Answer from the drawing. Dimensions are ordinates in mm from the lowest x, y and z of the part. A direction names the side the tool comes from. Give positions to 0.01 mm unless a question says otherwise; leave off trailing zeros. Write each loop counter-clockwise with the first axis right and the second up, starting at its lowest first coordinate (ties: lowest second). Pieces come first, ordered by that corner, then holes. Notation, with made-up numbers: (41, 13) -> (90, 13) arc R25 ccw to (90, 27) -> close; hole circle Ø4 at (-19, 52.25). An arc over 180 degrees is marked (long way). Use a Markdown table: item, result. Add a question column.
Q1. For the marked faces 3 and 4, determine the directions among +Z, -Z, +X, -X, +Y, -Y from which every point of the face is accessible in a straight line to the end or side of a thin tool.
Q2. Section D-D, the plane z = 36.5 is taken. Give the vertices of the cut face in (x, y).
Q3. Each of these flat-tipped pins is pushed along its axis until it touches: pin 1 Ø2.5 at (x, z) = (3.5, 25.5) entering from +Y; pin 2 Ø8 at (x, z) = (30.5, 22.5) entering from +Y; pin 3 Ø2 at (y, z) = (1, 36) entering from +X. Where does it stop, or does it pass through?
Q4. Section A-A, the plane x = 47.5 is taken. Give the vertices of the cut face in (y, z), plus the area to 3 significant figures.
Q5. For a pull along X with two mould halves and no side action, classify the marked faces 1 and 2 as pulls with the +X half, pulls with the -X half, needs draft (parallel to the pull), parting line crosses it, or undercut.
Q6. Section C-C, the plane y = 2 is taken. Give the vertices of the cut face in (x, z).
Q7. Consider line 1 (X direction, y = 3.1, z = 47.5); line 2 (X direction, y = 2.05, z = 22.5). Determine where each line is inside the solid, lowest interval first.
Q8. Section B-B, the plane z = 47.5 is taken. Give the vertices of the cut face in (x, y).
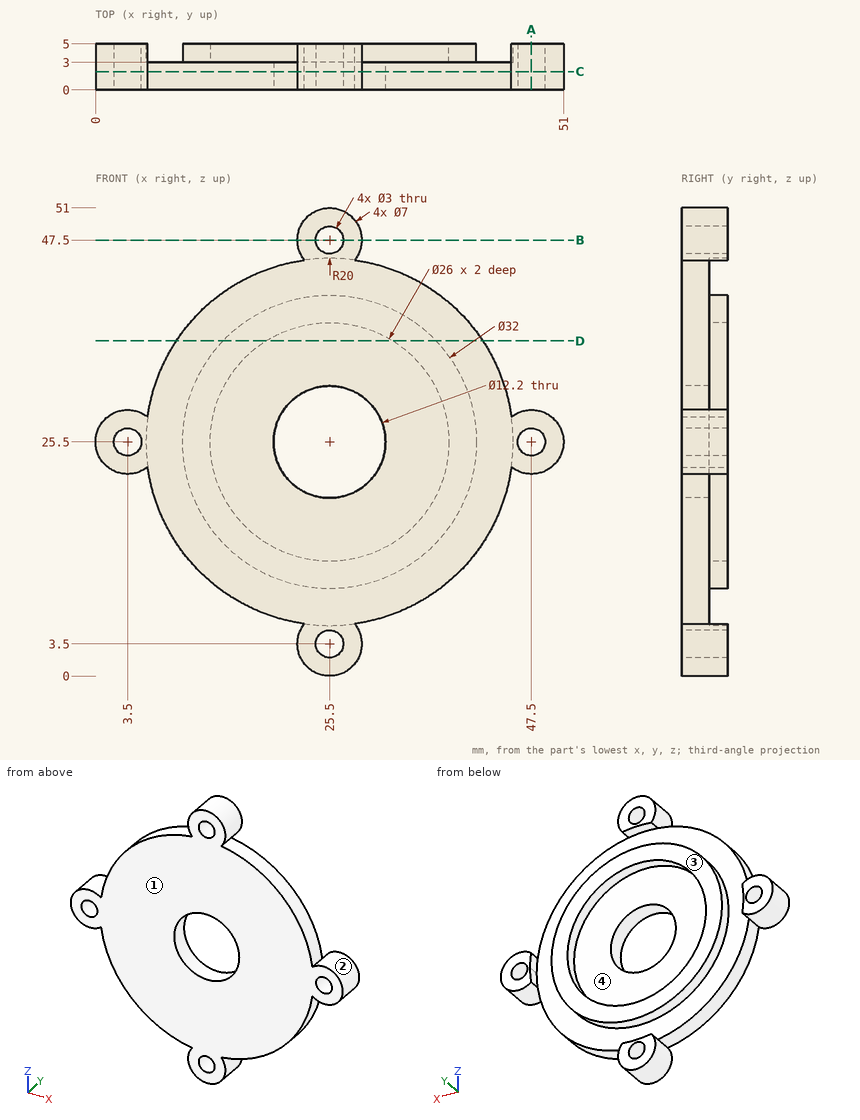
Result set:
| question | item | result |
|---|---|---|
| 1 | face 3 | +Z, -Z, +X, -X, +Y |
| 1 | face 4 | +Y |
| 2 | outline | (8.8, 0) -> (42.2, 0) -> (42.2, 3) -> (37.12, 3) -> (37.12, 5) -> (32.43, 5) -> (32.43, 3) -> (18.57, 3) -> (18.57, 5) -> (13.88, 5) -> (13.88, 3) -> (8.8, 3) -> close |
| 3 | pin 1 | passes through |
| 3 | pin 2 | stops at y = 3 |
| 3 | pin 3 | stops at x = 43.1 |
| 4 | outline | (0, 22) -> (5, 22) -> (5, 24) -> (0, 24) -> close; (0, 27) -> (5, 27) -> (5, 29) -> (0, 29) -> close |
| 4 | area | 20.0 mm2 |
| 5 | face 1 | needs draft |
| 5 | face 2 | undercut |
| 6 | outline | (5.69, 22.77) arc R20 ccw to (22.77, 5.69) arc R3.5 ccw (long way) to (28.23, 5.69) arc R20 ccw to (45.31, 22.77) arc R3.5 ccw (long way) to (45.31, 28.23) arc R20 ccw to (28.23, 45.31) arc R3.5 ccw (long way) to (22.77, 45.31) arc R20 ccw to (5.69, 28.23) arc R3.5 ccw (long way) to start; hole circle Ø3 at (3.5, 25.5); hole circle Ø12.2 at (25.5, 25.5); hole circle Ø3 at (25.5, 3.5); hole circle Ø3 at (25.5, 47.5); hole circle Ø3 at (47.5, 25.5) |
| 7 | line 1 | x = 22 to 24, 27 to 29 |
| 7 | line 2 | x = 1.7 to 5.3, 5.73 to 20.19, 30.81 to 45.27, 45.7 to 49.3 |
| 8 | outline | (22, 0) -> (24, 0) -> (24, 5) -> (22, 5) -> close; (27, 0) -> (29, 0) -> (29, 5) -> (27, 5) -> close |
